Input: dimensioned drawing with shaded views. Units: mm. Origin: part minimum x, y, z. A direction names the side the tool comes from. Round coordinates to 2 decimals unless told otherwise and drop trailing zeros. Order: outer loops, then holes, each group sorted by start corner. A loop starts at its lowest first (then second) coordinate and runs counter-clockwise, first axis right, second up. Notation, with made-up numbers: M 83.25,54 L 120.25,54 A33 cw 120.25,84 Z; hole C -13.75,-14.75 d8. An arc over 180 degrees is marked long. Use one line per item in the form item = value. Start each with the question number.
Q1. Material intervals for probe 1 along Y at (x, z) = (35, 3.45); probe 2 along Y at (x, z) = (26.5, 9); probe 3 along X at (y, z) = (14, 5.75), sorted ascending.
Q2. Section B-B (z = 8.5). Return the cut outline in (x, y).
Q3. Contact query for flat-ended pins moving along their axis: pin 1 (5 mm diameter, centred on x = 20, y = 10, fed in from +Z); pin 2 (1 mm diameter, centred on x = 10, z = 8.5, fed in from -Y); pin 3 (5 mm diameter, centred on x = 14, y = 12, fed in from +Z). Output: stop coordinate, or through.
Q4. Section D-D (y = 2.25). Return the cut outline in (x, z), plus the area to 4 significant figures.
Q5. Section C-C (x = 33.5). Return the cut outline in (y, z).
Q6. Reachability of the marked faces 5 and 6 from +Z, -Z, +X, -X, +Y, -Y: full face, straight path, thin tool, end or side. Return the list, or none.
Q7. Pull-direction query (X, two-part tool) for the marked faces 1, 2, 3 and 4; classes: pulls with the +X half, pulls with the -X half, needs draft (parallel to the pull), parting line crosses it, or undercut.
Q8. Section A-A (y = 10). Return the cut outline in (x, z), plus the area to 4 significant figures.
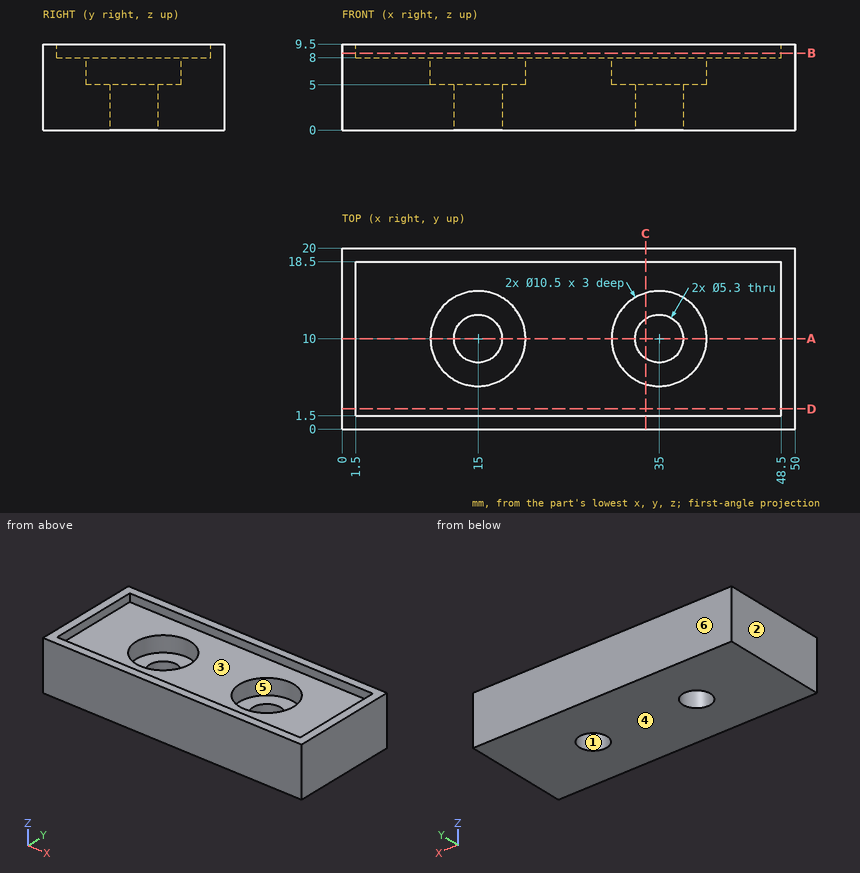
Results list:
q1.probe_1 = 0 to 7.35, 12.65 to 20
q1.probe_2 = 0 to 1.5, 18.5 to 20
q1.probe_3 = 0 to 11.6, 18.4 to 31.6, 38.4 to 50
q2.outline = M 0,0 L 50,0 L 50,20 L 0,20 Z; hole M 1.5,1.5 L 48.5,1.5 L 48.5,18.5 L 1.5,18.5 Z
q3.pin_1 = 8
q3.pin_2 = 0
q3.pin_3 = 5
q4.outline = M 0,0 L 50,0 L 50,9.5 L 48.5,9.5 L 48.5,8 L 1.5,8 L 1.5,9.5 L 0,9.5 Z
q4.area = 404.5 mm2
q5.outline = M 0,0 L 7.82,0 L 7.82,5 L 4.97,5 L 4.97,8 L 1.5,8 L 1.5,9.5 L 0,9.5 Z; M 12.18,0 L 20,0 L 20,9.5 L 18.5,9.5 L 18.5,8 L 15.03,8 L 15.03,5 L 12.18,5 Z
q6.face_5 = +Z
q6.face_6 = +Z, -Z, +X, -X, +Y
q7.face_1 = undercut
q7.face_2 = pulls with the -X half
q7.face_3 = undercut
q7.face_4 = needs draft
q8.outline = M 0,0 L 12.35,0 L 12.35,5 L 9.75,5 L 9.75,8 L 1.5,8 L 1.5,9.5 L 0,9.5 Z; M 17.65,0 L 32.35,0 L 32.35,5 L 29.75,5 L 29.75,8 L 20.25,8 L 20.25,5 L 17.65,5 Z; M 37.65,0 L 50,0 L 50,9.5 L 48.5,9.5 L 48.5,8 L 40.25,8 L 40.25,5 L 37.65,5 Z
q8.area = 288.5 mm2
